Geometry: final body of the model. Coordinates: model frame, mm. Face numbers are marked on the shaded views. A direction names the side the tool comes from. Give positions to 0.01 mm unless a question says otherwise; leave off trailing zeros. Write each loop counter-clockwise with the first axis right and the second up, starting at its lowest first coordinate (ties: lowest second). Pieces come first, ordered by that corner, then holes. Notation, with made-up numbers: (-0.75, 29) -> (36.25, 29) arc R23 ccw to (36.25, 52) -> close; hole circle Ø10 at (17.5, 73). An arc over 180 degrees is marked (long way). Answer in a Markdown table with one row per item. Add a question column.
Item 1: Section query A-A on y = 44. Output: boundary loops of the cut face in (x, z), plus the area to 3 significant figures.
Item 2: Draft query along Y for the marked faces 5, 6 and 7. Return one class per face: +Y half, -Y half, draft (parallel to the pull), parting line (faces both ways), or undercut.
Item 3: First-contact query: P1, Ø3, axis at x = -51.5, y = 17.5, coming from the +Z side; P2, Ø10, axis at x = -5, y = 15.5, coming from the -Z side; P3, Ø5.5, axis at y = 2.5, z = 32.5, coming from the +X side. Flat tips, straight axial feed; report the tip coordinate or a pass-through.
Item 4: Section query C-C on x = -42. Output: boundary loops of the cut face in (y, z).
Item 5: Material intervals for probe 1 along X at (y, z) = (65, 28); probe 2 along Z at (x, y) = (23.5, 72); probe 3 along Y at (x, z) = (95, -30), sorted ascending. Write a range as from..to.
Item 6: Section query B-B on z = 0. Output: boundary loops of the cut face in (x, y).
Item 7: Access query for the marked faces 1, 2, 3 and 4. Directions: +Z, -Z, +X, -X, +Y, -Y. A direction counts if a zero-diameter tool reaches every point of the face in a straight line with its end or side. Return the directions, or none.
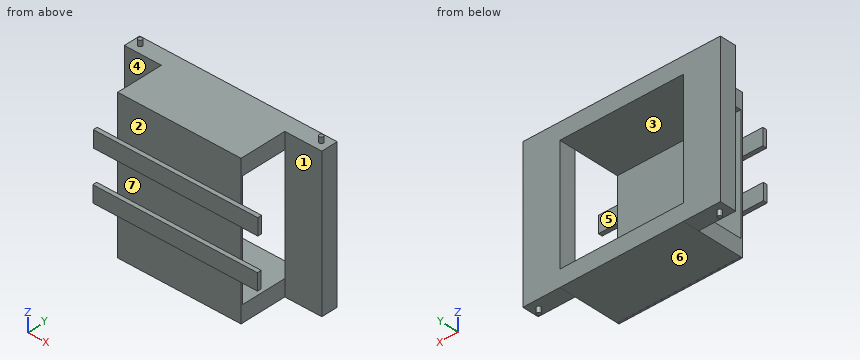
Autodesk Inventor part; units mm, degrees
ref_plane "YZ Plane" through (0, 0, 0) normal (1, 0, 0) x (0, 1, 0)
ref_plane "XZ Plane" through (0, 0, 0) normal (0, 1, 0) x (-1, 0, 0)
ref_plane "XY Plane" through (0, 0, 0) normal (0, 0, 1) x (1, 0, 0)
sketch "Эскиз1" plane through (0, 0, 0) normal (0, 1, 0) x (-1, 0, 0)
  line L0 (100.4756, 42.2222) -> (-99.5244, 42.2222)
  line L1 (-99.5244, 42.2222) -> (-99.5244, 22.2222)
  line L2 (-99.5244, 22.2222) -> (100.4756, 22.2222)
  line L3 (100.4756, 22.2222) -> (100.4756, 42.2222)
  line L4 (101, -17.7778) -> (-99, -17.7778)
  line L5 (-99, -17.7778) -> (-99, -37.7778)
  line L6 (-99, -37.7778) -> (101, -37.7778)
  line L7 (101, -37.7778) -> (101, -17.7778)
  point P0 (0, 0)
  dimension "d0" = 200
  dimension "d1" = 20
  dimension "d2" = 200
  dimension "d3" = 20
  dimension "d4" = 40
extrude "Выдавливание1" add sketch "Эскиз1" along normal blind 5
sketch "Эскиз2" plane through (0, 5, 0) normal (0, 1, 0) x (1, 0, 0)
  line L0 (-75.4756, -92.2222) -> (74.5244, -92.2222)
  line L1 (74.5244, -92.2222) -> (74.5244, 87.7778)
  line L2 (74.5244, 87.7778) -> (-75.4756, 87.7778)
  line L3 (-75.4756, 87.7778) -> (-75.4756, -92.2222)
  line L4 (-100.4756, -42.2222) -> (99.5244, -42.2222)
  line L5 (99.5244, -42.2222) -> (99.5244, -22.2222)
  line L6 (-100.4756, -22.2222) -> (-100.4756, -42.2222)
  point P0 (0, 0)
  dimension "d7" = 180
  dimension "d8" = 50
  dimension "d11" = 150
  dimension "d12" = 25
extrude "Выдавливание2" add sketch "Эскиз2" along normal blind 2
sketch "Эскиз3" plane through (0, 7, 0) normal (0, 1, 0) x (1, 0, 0)
  line L0 (-75.4756, 87.7778) -> (-75.4756, -92.2222)
  line L1 (74.5244, -92.2222) -> (74.5244, 87.7778)
  line L2 (-75.4756, -92.2222) -> (74.5244, -92.2222)
  line L3 (74.5244, -92.2222) -> (74.5244, -72.2222)
  line L4 (74.5244, -72.2222) -> (-75.4756, -72.2222)
  line L5 (-75.4756, -72.2222) -> (-75.4756, -92.2222)
  line L6 (-75.4756, 67.6742) -> (74.5244, 67.6742)
  line L7 (74.5244, 67.6742) -> (74.5244, 87.6742)
  line L8 (74.5244, 87.6742) -> (-75.4756, 87.6742)
  line L9 (-75.4756, 87.6742) -> (-75.4756, 67.6742)
  point P0 (0, 0)
  point P1 (-75.4756, 87.6742)
  dimension "d14" = 20
  dimension "d15" = 20
extrude "Выдавливание3" add sketch "Эскиз3" along normal blind 75 contours L8 L1 L6 L0 | L4 L1 L2 L0
sketch "Эскиз4" plane through (74.5244, 5, 92.2222) normal (1, 0, 0) x (0, 0, -1)
  line L0 (0, 77) -> (20, 77)
  line L1 (179.8965, 2) -> (179.8965, 77)
  line L2 (0, 77) -> (179.8965, 77)
  line L3 (179.8965, 77) -> (179.8965, 57)
  line L4 (179.8965, 57) -> (0, 57)
  line L5 (0, 57) -> (0, 77)
  point P0 (92.2222, -5)
  dimension "d18" = 20
extrude "Выдавливание4" add sketch "Эскиз4" along normal blind 45
sketch "Эскиз5" plane through (-75.4756, 5, -87.7778) normal (-1, 0, 0) x (0, 0, 1)
  line L0 (0.1035, 57) -> (0.1035, 77)
  line L1 (180, 0) -> (180, 57)
  line L2 (0.1035, 77) -> (180, 77)
  line L3 (180, 77) -> (180, 57)
  line L4 (180, 57) -> (0.1035, 57)
  line L5 (0.1035, 57) -> (0.1035, 77)
  point P0 (87.7778, -5)
extrude "Выдавливание5" add sketch "Эскиз5" along normal blind 45
sketch "Эскиз6" plane through (74.5244, 7, -87.6742) normal (0, 0, -1) x (-1, 0, 0)
  circle A0 centre (185, 65) radius 2.5
  line L0 (195, 75) -> (195, 55)
  circle A1 centre (-35, 65) radius 2.5
  line L1 (-45, 55) -> (-45, 75)
  line L2 (195, 75) -> (-45, 75)
  point P0 (74.5244, -7)
  dimension "d23" = 10
  dimension "d24" = 5
  dimension "d25" = 5
  dimension "d26" = 10
  dimension "d27" = 10
  dimension "d28" = 10
extrude "Выдавливание6" add sketch "Эскиз6" along normal blind 3
sketch "Эскиз7" plane through (-75.4756, 5, 92.2222) normal (0, 0, 1) x (1, 0, 0)
  circle A0 centre (-35, 67) radius 2.5
  circle A1 centre (-35, 67) radius 2.5
  circle A2 centre (185, 67) radius 2.5
  circle A3 centre (185, 67) radius 2.5
  point P0 (75.4756, -5)
extrude "Выдавливание7" add sketch "Эскиз7" along normal blind 3
sketch "Эскиз9" plane through (109.5244, 72, -90.6742) normal (0, 0, -1) x (-1, 0, 0)
  circle A0 centre (0, 0) radius 2.5
  circle A1 centre (0, 0) radius 2.5
  circle A2 centre (220, 0) radius 2.5
  circle A3 centre (220, 0) radius 2.5
  point P0 (109.5244, -72)
extrude "Выдавливание8" add sketch "Эскиз9" along normal blind 4
sketch "Эскиз10" plane through (-75.4756, 5, 92.2222) normal (0, 0, 1) x (1, 0, 0)
  circle A0 centre (-35, 67) radius 2.5
  circle A1 centre (-35, 67) radius 2.5
  circle A2 centre (185, 67) radius 2.5
  circle A3 centre (185, 67) radius 2.5
  point P0 (75.4756, -5)
extrude "Выдавливание9" add sketch "Эскиз10" along normal blind 7
properties part number "часть транспортера" material "Железо, ковкое"
Findings below:
| question | item | result |
|---|---|---|
| 1 | outline | (-75.48, -87.67) -> (74.52, -87.67) -> (74.52, -67.67) -> (-75.48, -67.67) -> close; (-75.48, 72.22) -> (74.52, 72.22) -> (74.52, 92.22) -> (-75.48, 92.22) -> close |
| 1 | area | 6,000 mm^2 |
| 2 | face 5 | undercut |
| 2 | face 6 | draft |
| 2 | face 7 | -Y half |
| 3 | P1 | stops at z = 92.22 |
| 3 | P2 | stops at z = -87.67 |
| 3 | P3 | stops at x = 99.52 |
| 4 | outline | (0, -37.78) -> (5, -37.78) -> (5, -87.78) -> (7, -87.78) -> (7, -87.67) -> (82, -87.67) -> (82, -67.67) -> (7, -67.67) -> (7, 72.22) -> (82, 72.22) -> (82, 92.22) -> (5, 92.22) -> (5, 42.22) -> (0, 42.22) -> (0, 22.22) -> (5, 22.22) -> (5, -17.78) -> (0, -17.78) -> close |
| 5 | probe 1 | x = -120.48..-75.48, 74.52..119.52 |
| 5 | probe 2 | z = -87.67..-67.67, 72.22..92.22 |
| 5 | probe 3 | y = 0..5, 62..82 |
| 6 | outline | (-120.48, 62) -> (-75.48, 62) -> (-75.48, 82) -> (-120.48, 82) -> close; (-75.48, 5) -> (74.52, 5) -> (74.52, 7) -> (-75.48, 7) -> close; (74.52, 62) -> (119.52, 62) -> (119.52, 82) -> (74.52, 82) -> close |
| 7 | face 1 | +Z, -Z, +X |
| 7 | face 2 | +Z, +X, -X, -Y |
| 7 | face 3 | +Y |
| 7 | face 4 | +Z, -Z, -X |
